```python
from build123d import *

# Parameters (mm, degrees)
F0_W     = 38.1
F0_H     = 38.1
F1_DEPTH = 38.1
F4_DEPTH = 38.1
F5_W     = 28.191894
F5_H     = 28.831113
F6_DEPTH = 38.1


with BuildPart() as f1:
    # F0 (on Front) → F1 (new body)
    with BuildSketch(Plane.XZ):
        with Locations((19.05, 19.05)):
            Rectangle(F0_W, F0_H)
    extrude(amount=F1_DEPTH)

    # F3 (on face) → F4 (cut)
    with BuildSketch(Plane.YZ.offset(38.1)):
        Polygon((0, 23.742571), (0, 31.250443), (-23.93651, 31.250443), (-23.93651, 23.93651), align=None)
        Polygon((0, 7.535568), (0, 15.957672), (-23.936734, 16.151613), (-23.936734, 7.535568), (0, 7.456388), align=None)
    extrude(amount=-F4_DEPTH, mode=Mode.SUBTRACT)

    # F5 (on offset) → F6 (cut)
    with BuildSketch(Plane.XZ.offset(38.1)):
        with Locations((14.095947, 23.684444)):
            Rectangle(F5_W, F5_H)
    extrude(amount=-F6_DEPTH, mode=Mode.SUBTRACT)


solid = f1.part
```
Here's how the part is built. I have some questions about the finished solid (model axes, mm). A direction names the side the tool comes from. Give positions to 0.01 mm unless a question says otherwise; leave off trailing zeros. Order: outer loops, then holes, each group sorted by start corner. A loop starts at its lowest first (then second) coordinate and runs counter-clockwise, first axis right, second up. Notation, with made-up numbers: (18.5, 38) -> (55.5, 38) arc R31 cw to (55.5, 66) -> close; hole circle Ø2 at (-13.5, 80.25). An arc over 180 degrees is marked (long way). Use CSV: the item, a comma, the result in double quotes. Start each with the question number.
Item 1: Thinking about a two-plate mould opening in Z: for faces 4 (the flat face through (33, -23.937, 28)), 5 (the flat face through (33, 0, 35)), 6 (the flat face through (33, -19, 38.1)), which applies, pulls with the +Z half, pulls with the -Z half, needs draft (parallel to the pull), parting line crosses it, or undercut?
Item 2: If I drill on probe 1 along Z at (x, y) = (26, -24); probe 2 along X at (y, z) = (-26, 20); probe 3 along Z at (x, y) = (31.5, -4), over which ranges is the centre line in solid material (lowest first)? Write a range as [from, to].
Item 3: Suppose I cut it at B-B (x = 32). List the corners of the cut face in (y, z) for me, and give its area (3 significant figures).
Item 4: Suppose I cut it at A-A (y = -5). List the corners of the cut face in (x, z) for me.
Item 5: Suppose I cut it at D-D (y = -20). List the corners of the cut face in (x, z) for me.
Item 6: Suppose I cut it at C-C (z = 28). List the corners of the cut face in (x, y) for me.
Item 7: I'm going to push a flat-ended pin straight in: P1, Ø8, axis at x = 7, y = -25, coming from the +Z side. Where does the tip first touch, or does it pass through?
Item 8: On a 3-axis mill with a long thin cutter (end or side, diameter ignored), from which of +Z, -Z, +X, -X, +Y, -Y can I reach the whole of each face in a straight line? I mean faces 1 (the flat face through (33, -12, 31.25)), 2 (the flat face through (14, -31, 9.269)), 3 (the flat face through (38.1, -19, 19)). Say none if no direction works.
Answer block:
1,face 4,"undercut"
1,face 5,"needs draft"
1,face 6,"pulls with the +Z half"
2,probe 1,"z = [0, 9.27]"
2,probe 2,"x = [28.19, 38.1]"
2,probe 3,"z = [0, 7.47], [15.99, 23.77], [31.25, 38.1]"
3,outline,"(-38.1, 0) -> (0, 0) -> (0, 7.46) -> (-23.94, 7.54) -> (-23.94, 16.15) -> (0, 15.96) -> (0, 23.74) -> (-23.94, 23.94) -> (-23.94, 31.25) -> (0, 31.25) -> (0, 38.1) -> (-38.1, 38.1) -> close"
3,area,"1,070 mm^2"
4,outline,"(0, 0) -> (38.1, 0) -> (38.1, 7.47) -> (0, 7.47) -> close; (28.19, 16) -> (38.1, 16) -> (38.1, 23.78) -> (28.19, 23.78) -> close; (28.19, 31.25) -> (38.1, 31.25) -> (38.1, 38.1) -> (28.19, 38.1) -> close"
5,outline,"(0, 0) -> (38.1, 0) -> (38.1, 7.52) -> (0, 7.52) -> close; (28.19, 16.12) -> (38.1, 16.12) -> (38.1, 23.9) -> (28.19, 23.9) -> close; (28.19, 31.25) -> (38.1, 31.25) -> (38.1, 38.1) -> (28.19, 38.1) -> close"
6,outline,"(28.19, -38.1) -> (38.1, -38.1) -> (38.1, -23.94) -> (28.19, -23.94) -> close"
7,P1,"stops at z = 9.27"
8,face 1,"+X, -X, +Y"
8,face 2,"+Z, -X, +Y, -Y"
8,face 3,"+Z, -Z, +X, +Y, -Y"
